Input: part model. Units: mm. Frame: model coordinates. Face numbers are marked on the shaded views. A direction names the side the tool comes from. Give positions to 0.01 mm unless a question says otherwise; leave off trailing zeros. Loops run counter-clockwise (first coordinate to the right, second up) from the corner with the lowest first, then second, coordinate; pieces in that order, holes last. Notation, with made-up numbers: (-33, -1.75) -> (26, -1.75) arc R24 cw to (26, 31.25) -> close; hole circle Ø6 at (-19.75, -23.75). An arc over 180 degrees is marked (long way). Use CSV: the item, a comma, the result in double quotes.
```python
from build123d import *

# Parameters (mm, degrees)
CROQUIS1_R                   = 17.5
CROQUIS1_R_2                 = 1.65
SALIENTE_EXTRUIR1_DEPTH      = 3.5
CORTAR_EXTRUIR1_DEPTH        = 2.5
CROQUIS4_R                   = 3.6
CORTAR_EXTRUIR2_DEPTH        = 25.874685928
CORTAR_EXTRUIR2_DEPTH_BACK   = 25.874685928
CROQUIS5_R                   = 5.6
CROQUIS5_R_2                 = 3.6
SALIENTE_EXTRUIR2_DEPTH      = 1.7
SALIENTE_EXTRUIR3_REACH      = 52.742
SALIENTE_EXTRUIR3_END_RADIUS = 17.5
CROQUIS6_W                   = 25
CROQUIS6_H                   = 3.5
CROQUIS7_W                   = 25
CROQUIS7_H                   = 5
SALIENTE_EXTRUIR4_DEPTH      = 35
REDONDEO1_R                  = 3.5
REDONDEO1_OF_SIMETR_A1_R     = 3.5
CHAFL_N1_SIZE                = 0.254
CORTAR_EXTRUIR3_DEPTH        = 2.5
CROQUIS10_R                  = 10.15
CROQUIS10_R_2                = 1.425
CROQUIS10_R_3                = 1
CORTAR_EXTRUIR7_DEPTH        = 2
CORTAR_EXTRUIR8_REACH        = 71.379
CROQUIS11_R                  = 4.65
CORTAR_EXTRUIR9_REACH        = 73.781
CROQUIS13_R                  = 1.425
REDONDEO2_R                  = 10
CORTAR_EXTRUIR10_DEPTH       = 2.5


with BuildPart() as part:
    # Croquis1 → Saliente-Extruir1 (new body)
    with BuildSketch(Plane(origin=(0, 0, 0), x_dir=(1, 0, 0), z_dir=(0, 1, 0))):
        with Locations(Location((0, 0, 0), (0, 0, 270))):
            Circle(CROQUIS1_R)
        with Locations(Location((0, 0, 0), (0, 0, 270))):
            Circle(CROQUIS1_R_2, mode=Mode.SUBTRACT)
        with BuildLine():
            Line((-1.997159934, -12.106546701), (-2.53, -2.118749631))
            ThreePointArc((-2.53, -2.118749631), (-3.3, 0), (-2.53, 2.118749631))
            Line((-2.53, 2.118749631), (-1.997159934, 12.106546701))
            ThreePointArc((-1.997159934, 12.106546701), (0, 14), (1.997159934, 12.106546701))
            Line((1.997159934, 12.106546701), (2.53, 2.118749631))
            ThreePointArc((2.53, 2.118749631), (3.3, 0), (2.53, -2.118749631))
            Line((2.53, -2.118749631), (1.997159934, -12.106546701))
            ThreePointArc((1.997159934, -12.106546701), (0, -14), (-1.997159934, -12.106546701))
        make_face()
        with Locations(Location((0, 0, 0), (0, 0, 270))):
            Circle(CROQUIS1_R_2, mode=Mode.SUBTRACT)
    extrude(amount=SALIENTE_EXTRUIR1_DEPTH)

    # Croquis2 → Cortar-Extruir1 (cut)
    with BuildSketch(Plane(origin=(0, 3.5, 0), x_dir=(1, 0, 0), z_dir=(0, 1, 0))):
        with BuildLine():
            Line((-1.997159934, -12.106546701), (-2.53, -2.118749631))
            ThreePointArc((-2.53, -2.118749631), (-3.3, 0), (-2.53, 2.118749631))
            Line((-2.53, 2.118749631), (-1.997159934, 12.106546701))
            ThreePointArc((-1.997159934, 12.106546701), (0, 14), (1.997159934, 12.106546701))
            Line((1.997159934, 12.106546701), (2.53, 2.118749631))
            ThreePointArc((2.53, 2.118749631), (3.3, 0), (2.53, -2.118749631))
            Line((2.53, -2.118749631), (1.997159934, -12.106546701))
            ThreePointArc((1.997159934, -12.106546701), (0, -14), (-1.997159934, -12.106546701))
        make_face()
    extrude(amount=-CORTAR_EXTRUIR1_DEPTH, mode=Mode.SUBTRACT)

    # Croquis4 → Cortar-Extruir2 (cut, two sides)
    with BuildSketch(Plane(origin=(0, 1, 0), x_dir=(1, 0, 0), z_dir=(0, 1, 0))) as cortar_extruir2_sk:
        with Locations(Location((0, 0, 0), (0, 0, 270))):
            Circle(CROQUIS4_R)
    extrude(amount=CORTAR_EXTRUIR2_DEPTH, mode=Mode.SUBTRACT)
    extrude(cortar_extruir2_sk.sketch, amount=-CORTAR_EXTRUIR2_DEPTH_BACK, mode=Mode.SUBTRACT)

    # Croquis5 → Saliente-Extruir2 (add)
    with BuildSketch(Plane.XZ):
        with Locations(Location((0, 0, 0), (0, 0, 90))):
            Circle(CROQUIS5_R)
        with Locations(Location((0, 0, 0), (0, 0, 90))):
            Circle(CROQUIS5_R_2, mode=Mode.SUBTRACT)
    extrude(amount=SALIENTE_EXTRUIR2_DEPTH)

    # Saliente-Extruir3: up to this cylinder (the profile starts outside it)
    saliente_extruir3_end = Plane(origin=(0, 1.75, 0), z_dir=(0, -1, 0)) * Cylinder(SALIENTE_EXTRUIR3_END_RADIUS, 141.484, mode=Mode.PRIVATE)
    # Croquis6 → Saliente-Extruir3 (add, up to the surface)
    with BuildSketch(Plane.XY.offset(30), mode=Mode.PRIVATE) as saliente_extruir3_sk1:
        with Locations((0, 1.75)):
            Rectangle(CROQUIS6_W, CROQUIS6_H)
    saliente_extruir3_tool1 = extrude(saliente_extruir3_sk1.sketch, amount=-SALIENTE_EXTRUIR3_REACH, mode=Mode.PRIVATE) - saliente_extruir3_end
    saliente_extruir3 = saliente_extruir3_tool1.solids().sort_by_distance((0, 1.75, 30))[0]
    add(saliente_extruir3)

    # Croquis7 → Saliente-Extruir4 (add)
    with BuildSketch(Plane(origin=(0, 3.5, 0), x_dir=(1, 0, 0), z_dir=(0, 1, 0))):
        with Locations((0, -27.5)):
            Rectangle(CROQUIS7_W, CROQUIS7_H)
    saliente_extruir4 = extrude(amount=SALIENTE_EXTRUIR4_DEPTH)

    # Redondeo1
    redondeo1_edges = [part.edges().sort_by_distance(p)[0] for p in [
        (0, 0, 30),
        (0, 3.5, 25),
    ]]
    fillet(redondeo1_edges, radius=REDONDEO1_R)

    # Simetría1: Saliente-Extruir3, Saliente-Extruir4 across plane
    add(saliente_extruir3.mirror(Plane.XY))
    add(saliente_extruir4.mirror(Plane.XY))

    # Redondeo1 of Simetría1
    redondeo1_of_simetr_a1_edges = [part.edges().sort_by_distance(p)[0] for p in [
        (0, 0, -30),
        (0, 3.5, -25),
    ]]
    fillet(redondeo1_of_simetr_a1_edges, radius=REDONDEO1_OF_SIMETR_A1_R)

    # Chaflán1
    chafl_n1_edges = [part.edges().sort_by_distance(p)[0] for p in [
        (0, -1.7, -3.6),
    ]]
    chamfer(chafl_n1_edges, length=CHAFL_N1_SIZE)

    # Croquis8 → Cortar-Extruir3 (cut)
    with BuildSketch(Plane(origin=(0, 3.5, 0), x_dir=(1, 0, 0), z_dir=(0, 1, 0))):
        with BuildLine():
            Line((-2.795512377, -2.719395254), (-2.374256235, -12.106546701))
            ThreePointArc((-2.374256235, -12.106546701), (0, -14.376645718), (2.374256235, -12.106546701))
            Line((2.374256235, -12.106546701), (2.795512377, -2.719395254))
            ThreePointArc((2.795512377, -2.719395254), (3.9, 0), (2.795512377, 2.719395254))
            Line((2.795512377, 2.719395254), (2.374256235, 12.106546701))
            ThreePointArc((2.374256235, 12.106546701), (0, 14.376645718), (-2.374256235, 12.106546701))
            Line((-2.374256235, 12.106546701), (-2.795512377, 2.719395254))
            ThreePointArc((-2.795512377, 2.719395254), (-3.9, 0), (-2.795512377, -2.719395254))
        make_face()
    extrude(amount=-CORTAR_EXTRUIR3_DEPTH, mode=Mode.SUBTRACT)

    # Croquis10 → Cortar-Extruir7 (cut)
    with BuildSketch(Plane(origin=(0, 0, 30), x_dir=(-1, 0, 0), z_dir=(0, 0, -1))):
        with Locations(Location((0, 26.5, 0), (0, 0, 180))):
            Circle(CROQUIS10_R)
        with Locations((-7, 26.5)):
            Circle(CROQUIS10_R_2, mode=Mode.SUBTRACT)
        with Locations((0, 33.5)):
            Circle(CROQUIS10_R_2, mode=Mode.SUBTRACT)
        with Locations((0, 26.5)):
            Circle(CROQUIS10_R_3, mode=Mode.SUBTRACT)
        with Locations((7, 26.5)):
            Circle(CROQUIS10_R_2, mode=Mode.SUBTRACT)
        with Locations((0, 19.5)):
            Circle(CROQUIS10_R_2, mode=Mode.SUBTRACT)
        with Locations((7, 26.5)):
            Circle(CROQUIS10_R_2)
        with Locations((0, 26.5)):
            Circle(CROQUIS10_R_3)
        with Locations((0, 33.5)):
            Circle(CROQUIS10_R_2)
        with Locations((-7, 26.5)):
            Circle(CROQUIS10_R_2)
        with Locations((0, 19.5)):
            Circle(CROQUIS10_R_2)
    cortar_extruir7 = extrude(amount=CORTAR_EXTRUIR7_DEPTH, mode=Mode.SUBTRACT)

    # Croquis11 → Cortar-Extruir8 (cut, up to next)
    with BuildSketch(Plane(origin=(0, 0, 25), x_dir=(-1, 0, 0), z_dir=(0, 0, -1)), mode=Mode.PRIVATE) as cortar_extruir8_sk1:
        with Locations((0, 26.5)):
            Circle(CROQUIS11_R)
    cortar_extruir8_tool1 = extrude(cortar_extruir8_sk1.sketch, amount=-CORTAR_EXTRUIR8_REACH, mode=Mode.PRIVATE) & part.part
    cortar_extruir8 = cortar_extruir8_tool1.solids().sort_by_distance((0, 26.5, 25))[0]
    add(cortar_extruir8, mode=Mode.SUBTRACT)

    # Croquis13 → Cortar-Extruir9 (cut, up to next)
    with BuildSketch(Plane.XY.offset(28), mode=Mode.PRIVATE) as cortar_extruir9_sk1:
        with Locations((0, 19.5)):
            Circle(CROQUIS13_R)
    cortar_extruir9_tool1 = extrude(cortar_extruir9_sk1.sketch, amount=-CORTAR_EXTRUIR9_REACH, mode=Mode.PRIVATE) & part.part
    # Croquis13 → Cortar-Extruir9 (cut, up to next)
    with BuildSketch(Plane.XY.offset(28), mode=Mode.PRIVATE) as cortar_extruir9_sk2:
        with Locations((7, 26.5)):
            Circle(CROQUIS13_R)
    cortar_extruir9_tool2 = extrude(cortar_extruir9_sk2.sketch, amount=-CORTAR_EXTRUIR9_REACH, mode=Mode.PRIVATE) & part.part
    # Croquis13 → Cortar-Extruir9 (cut, up to next)
    with BuildSketch(Plane.XY.offset(28), mode=Mode.PRIVATE) as cortar_extruir9_sk3:
        with Locations((0, 33.5)):
            Circle(CROQUIS13_R)
    cortar_extruir9_tool3 = extrude(cortar_extruir9_sk3.sketch, amount=-CORTAR_EXTRUIR9_REACH, mode=Mode.PRIVATE) & part.part
    # Croquis13 → Cortar-Extruir9 (cut, up to next)
    with BuildSketch(Plane.XY.offset(28), mode=Mode.PRIVATE) as cortar_extruir9_sk4:
        with Locations((-7, 26.5)):
            Circle(CROQUIS13_R)
    cortar_extruir9_tool4 = extrude(cortar_extruir9_sk4.sketch, amount=-CORTAR_EXTRUIR9_REACH, mode=Mode.PRIVATE) & part.part
    cortar_extruir9_1 = cortar_extruir9_tool1.solids().sort_by_distance((0, 19.5, 28))[0]
    add(cortar_extruir9_1, mode=Mode.SUBTRACT)
    cortar_extruir9_2 = cortar_extruir9_tool2.solids().sort_by_distance((7, 26.5, 28))[0]
    add(cortar_extruir9_2, mode=Mode.SUBTRACT)
    cortar_extruir9_3 = cortar_extruir9_tool3.solids().sort_by_distance((0, 33.5, 28))[0]
    add(cortar_extruir9_3, mode=Mode.SUBTRACT)
    cortar_extruir9_4 = cortar_extruir9_tool4.solids().sort_by_distance((-7, 26.5, 28))[0]
    add(cortar_extruir9_4, mode=Mode.SUBTRACT)
    cortar_extruir9 = cortar_extruir9_1 + cortar_extruir9_2 + cortar_extruir9_3 + cortar_extruir9_4  # Cortar-Extruir9 as one shape, for the pattern or mirror that repeats it

    # Simetría2: Cortar-Extruir7, Cortar-Extruir8, Cortar-Extruir9 across plane
    add(cortar_extruir7.mirror(Plane.XY), mode=Mode.SUBTRACT)
    add(cortar_extruir8.mirror(Plane.XY), mode=Mode.SUBTRACT)
    add(cortar_extruir9.mirror(Plane.XY), mode=Mode.SUBTRACT)

    # Redondeo2
    redondeo2_edges = [part.edges().sort_by_distance(p)[0] for p in [
        (12.5, 38.5, -27.5),
        (-12.5, 38.5, -27.5),
        (12.5, 38.5, 27.5),
        (-12.5, 38.5, 27.5),
    ]]
    fillet(redondeo2_edges, radius=REDONDEO2_R)

    # Croquis15 → Cortar-Extruir10 (cut)
    with BuildSketch(Plane(origin=(0, 3.5, 0), x_dir=(1, 0, 0), z_dir=(0, 1, 0))):
        with BuildLine():
            Line((2.374256235, 12.106546701), (2.20456569, 15.887882306))
            ThreePointArc((2.20456569, 15.887882306), (0, 17.376645718), (-2.20456569, 15.887882306))
            Line((-2.20456569, 15.887882306), (-2.374256235, 12.106546701))
            ThreePointArc((-2.374256235, 12.106546701), (0, 14.376645718), (2.374256235, 12.106546701))
        make_face()
        with BuildLine():
            Line((2.374256235, -12.106546701), (2.20456569, -15.887882306))
            ThreePointArc((2.20456569, -15.887882306), (0, -17.376645718), (-2.20456569, -15.887882306))
            Line((-2.20456569, -15.887882306), (-2.374256235, -12.106546701))
            ThreePointArc((-2.374256235, -12.106546701), (0, -14.376645718), (2.374256235, -12.106546701))
        make_face()
    extrude(amount=-CORTAR_EXTRUIR10_DEPTH, mode=Mode.SUBTRACT)


solid = part.part
```
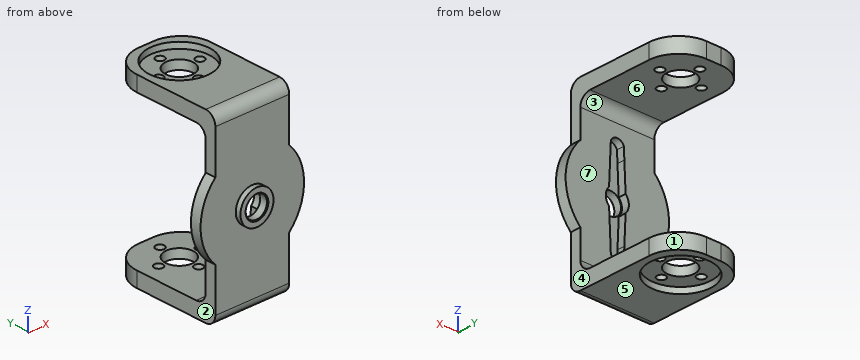
1) Mould query, pull axis Z, two halves, no side actions, for the marked faces 4, 5, 6 and 7. Classes: pulls with the +Z half, pulls with the -Z half, needs draft (parallel to the pull), parting line crosses it, or undercut.
From the geometry:
face 4,"needs draft"
face 5,"pulls with the -Z half"
face 6,"undercut"
face 7,"undercut"
2) Reachability of the marked faces 1, 2 and 3 from +Z, -Z, +X, -X, +Y, -Y: full face, straight path, thin tool, end or side. Return the list, or none.
From the geometry:
face 1,"+Z, -Z, +X, +Y"
face 2,"-Z, -X, +Y, -Y"
face 3,"+X, -X, +Y"
3) Ray query, line 1 (Y direction, x = 0, z = 26) (3 decimals); line 2 (Z direction, x = -5.5, y = 25); line 3 (X direction, y = 26, z = -27). Return the intervals inside material, ascending.
From the geometry:
line 1,"y = 0 to 18.075, 20.925 to 21.85, 31.15 to 32.075, 34.925 to 38.5"
line 2,"z = -28 to -25, 25 to 28"
line 3,"x = -12.5 to -8.33, -5.67 to -4.62, 4.62 to 5.67, 8.33 to 12.5"
4) Section query A-A (z = 0). Return loops of the section in (x, y).
From the geometry:
outline,"(-17.5, 0) -> (-5.6, 0) -> (-5.6, -1.7) -> (-3.85, -1.7) -> (-3.6, -1.45) -> (-3.6, 1) -> (-3.9, 1) -> (-3.9, 3.5) -> (-17.5, 3.5) -> close; (3.6, -1.45) -> (3.85, -1.7) -> (5.6, -1.7) -> (5.6, 0) -> (17.5, 0) -> (17.5, 3.5) -> (3.9, 3.5) -> (3.9, 1) -> (3.6, 1) -> close"
5) Section query B-B (y = 12). Return loops of the section in (x, z).
From the geometry:
outline,"(-12.5, -30) -> (12.5, -30) -> (12.5, -25) -> (-12.5, -25) -> close; (-12.5, 25) -> (12.5, 25) -> (12.5, 30) -> (-12.5, 30) -> close"
6) Contact query for flat-ended pins moving along their axis: pin 1 (4.5 mm diameter, centred on x = 7, y = 26.5, fed in from -Z); pin 2 (10 mm diameter, centred on x = 10.5, z = 11.5, fed in from -Y); pin 3 (19.5 mm diameter, centred on y = 19.5, z = -22, fed in from +X); pin 4 (7.5 mm diameter, centred on x = 0, y = 26.5, fed in from -Z). Output: stop coordinate, or through.
From the geometry:
pin 1,"stops at z = -28"
pin 2,"stops at y = 0"
pin 3,"stops at x = 12.5"
pin 4,"passes through"
7) Section query C-C (x = -7). Return loops of the section in (y, z) (3 decimals).
From the geometry:
outline,"(0, -26.5) arc R3.5 ccw to (3.5, -30) -> (19.15, -30) -> (19.15, -28) -> (25.075, -28) -> (25.075, -25) -> (7, -25) arc R3.5 cw to (3.5, -21.5) -> (3.5, 21.5) arc R3.5 cw to (7, 25) -> (25.075, 25) -> (25.075, 28) -> (19.15, 28) -> (19.15, 30) -> (3.5, 30) arc R3.5 ccw to (0, 26.5) -> close; (27.925, -28) -> (33.85, -28) -> (33.85, -30) -> (37.43, -30) -> (37.43, -25) -> (27.925, -25) -> close; (27.925, 25) -> (37.43, 25) -> (37.43, 30) -> (33.85, 30) -> (33.85, 28) -> (27.925, 28) -> close"
8) Section query D-D (y = 19.5). Return loops of the section in (x, z) (3 decimals).
From the geometry:
outline,"(-12.5, -30) -> (-7.35, -30) -> (-7.35, -28) -> (-1.425, -28) -> (-1.425, -25) -> (-12.5, -25) -> close; (-12.5, 25) -> (-1.425, 25) -> (-1.425, 28) -> (-7.35, 28) -> (-7.35, 30) -> (-12.5, 30) -> close; (1.425, -28) -> (7.35, -28) -> (7.35, -30) -> (12.5, -30) -> (12.5, -25) -> (1.425, -25) -> close; (1.425, 25) -> (12.5, 25) -> (12.5, 30) -> (7.35, 30) -> (7.35, 28) -> (1.425, 28) -> close"
